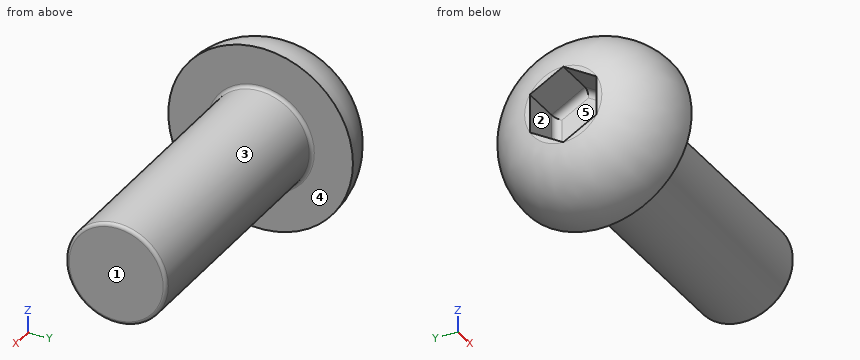
Autodesk Inventor part; units mm, degrees
ref_plane "YZ Plane" through (0, 0, 0) normal (1, 0, 0) x (0, 1, 0)
ref_plane "XZ Plane" through (0, 0, 0) normal (0, 1, 0) x (-1, 0, 0)
ref_plane "XY Plane" through (0, 0, 0) normal (0, 0, 1) x (1, 0, 0)
sketch "スケッチ1" plane through (0, 0, 0) normal (0, 0, 1) x (1, 0, 0)
  line L0 (0, 0) -> (8, 0)
  line L1 (8, 0) -> (8, 1.5)
  line L2 (8, 1.5) -> (0, 1.5)
  line L3 (0, 1.5) -> (0, 0)
  line L4 (0, 0) -> (0, 2.75)
  line L5 (0, 0) -> (-2, 0)
  line L6 (-2, 0) -> (0, 0)
  line L7 (-2, 0) -> (-2, 1.15)
  arc A0 (0, 2.75) -> (-2, 1.15) centre (-0.0403, 0.7504) ccw
  dimension "d0" = 1.5
  dimension "d1" = 8
  dimension "d3" = 2
  dimension "d4" = 2.75
  dimension "d5" = 1.15
  dimension "d6" = 2
revolve "回転1" add sketch "スケッチ1" angle 360 about axis through (-2, 0, 0) along (1, 0, 0)
thread "ねじ1"
sketch "スケッチ2" plane through (-2, 0, 0) normal (-1, 0, 0) x (0, 0, 1)
  circle A0 centre (0, 0) radius 1.15
  line L0 (-0.575, 0.9959) -> (0.575, 0.9959)
  line L1 (0.575, 0.9959) -> (1.15, 0)
  line L2 (1.15, 0) -> (0.575, -0.9959)
  line L3 (0.575, -0.9959) -> (-0.575, -0.9959)
  line L4 (-0.575, -0.9959) -> (-1.15, 0)
  line L5 (-1.15, 0) -> (-0.575, 0.9959)
  dimension "d10" = 1.15
  dimension "d11" = 1.9919
extrude "押し出し1" cut sketch "スケッチ2" against normal blind 1.4 contours L2 L3 L4 L5 L0 L1
fillet "フィレット1" radius 0.2 6 edges at (-0.6, 0.9959, 0) (-0.6, 0.498, 0.8625) (-0.6, 0.498, -0.8625) (-0.6, -0.498, -0.8625) (-0.6, -0.9959, 0) (-0.6, -0.498, 0.8625)
fillet "フィレット2" radius 0.1 1 edges at (0, -1.5, 0)
fillet "フィレット3" radius 0.1 1 edges at (8, -1.5, 0)
properties part number "ネジボタンM3L8" material "鋼"
Check sheet for the modelled part. Datum: model origin and axes. Units: mm. Face numbers are marked on the shaded views. A direction names the side the tool comes from. Round coordinates to 2 decimals unless told otherwise and drop trailing zeros. Loops run counter-clockwise (first coordinate to the right, second up) from the corner with the lowest first, then second, coordinate; pieces in that order, holes last.
1. Gauge pin test, flat ends, axial feed: pin 1 Ø3 at (x, y) = (-0.5, 1) entering from -Z; pin 2 Ø1.5 at (x, z) = (3, 0.5) entering from +Y; pin 3 Ø0.6 at (x, z) = (-1.5, 0) entering from +Y; pin 4 Ø2 at (x, y) = (4, -2) entering from +Z. Record the tip position at first contact, or that the pin passes through.
2. Scan lines: probe 1 along Z at (x, y) = (5.5, 0); probe 2 along X at (y, z) = (-1.8, -1.8); probe 3 along Y at (x, z) = (4.25, -0.7). Record each from-to range of solid material in increasing order.
3. Mould release check, pull along Y, two halves, no side actions. Record for the marked faces 3, 4 and 5: released by +Y, released by -Y, zero draft, split by the parting line, or undercut.
4. Set-up check for the marked faces 1 and 2: record each of +Z, -Z, +X, -X, +Y, -Y from which the full face is reachable in a straight line by a thin tool's end or side.
5. Sectioned sample at A-A on x = 1. Record the boundary of the cut face in (y, z).
Recorded:
1. pin 1: stops at z = -2.75
1. pin 2: stops at y = 1.5
1. pin 3: stops at y = 2.38
1. pin 4: stops at z = 1.12
2. probe 1: z = -1.5 to 1.5
2. probe 2: x = -0.92 to 0
2. probe 3: y = -1.33 to 1.33
3. face 3: split by the parting line
3. face 4: zero draft
3. face 5: undercut
4. face 1: +Z, -Z, +X, +Y, -Y
4. face 2: -X
5. outline: circle Ø3 at (0, 0)
